The drawing under review shows one solid part. Ordinate dimensions are in mm from its lowest x, y, z. A direction names the side the tool comes from. Coordinates: 2 decimals unless noted, no trailing zeros. Order: outer loops, then holes, each group sorted by start corner. A loop starts at its lowest first (then second) coordinate and runs counter-clockwise, first axis right, second up.
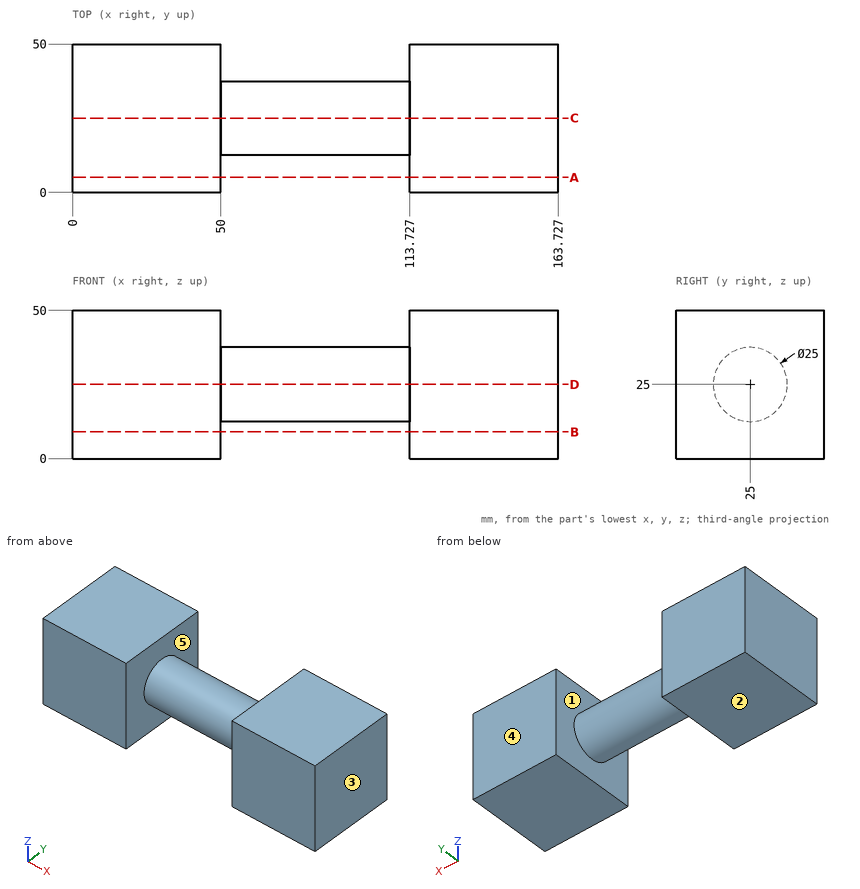
(1) Draft analysis for pull direction X (two halves, no side actions). For the marked faces 3, 4 and 5, state which applies: released by +X, released by -X, zero draft, split by the parting line, or undercut.
A:
face 3: released by +X
face 4: zero draft
face 5: undercut
(2) We need section C-C, the plane y = 25. Write out the cut boundary in (x, z).
A:
outline: (0, 0) - (50, 0) - (50, 12.5) - (113.73, 12.5) - (113.73, 0) - (163.73, 0) - (163.73, 50) - (113.73, 50) - (113.73, 37.5) - (50, 37.5) - (50, 50) - (0, 50) - close
(3) We need section A-A, the plane y = 5. Write out the cut boundary in (x, z), and give its area (3 significant figures).
A:
outline: (0, 0) - (50, 0) - (50, 50) - (0, 50) - close; (113.73, 0) - (163.73, 0) - (163.73, 50) - (113.73, 50) - close
area: 5,000 mm2
(4) Wall thickness on probe 1 along X at (y, z) = (45, 34); probe 2 along Y at (x, z) = (58, 33) (1 decimal); probe 3 along Z at (x, y) = (64, 30): over which ranges is each line inside the solid? List them lowest first.
A:
probe 1: x = 0 to 50, 113.73 to 163.73
probe 2: y = 15.4 to 34.6
probe 3: z = 13.54 to 36.46
(5) For pin 1 Ø1 at (x, z) = (110, 37) entering from -Y; pin 2 Ø1.5 at (x, z) = (108, 26) entering from -Y; pin 3 Ø8 at (x, y) = (109.5, 34) entering from -Z, all flat-tipped, find the tip position at first contact; note any pin that passes through.
A:
pin 1: stops at y = 20.1
pin 2: stops at y = 12.5
pin 3: stops at z = 13.54
(6) Machinability: for the marked faces 1 and 2, which of the approach directions +Z, -Z, +X, -X, +Y, -Y give a long, thin tool a straight path to every point of the face, cutting with its end or side? Answer none if there is none.
A:
face 1: none
face 2: -Z, +X, -X, +Y, -Y
